```python
from build123d import *

# Parameters (mm, degrees)
SKETCH1_W           = 24
SKETCH1_H           = 16
BOSS_EXTRUDE1_DEPTH = 10
SKETCH2_R           = 4.3
SKETCH2_R_2         = 1.6
CUT_EXTRUDE2_DEPTH  = 11


with BuildPart() as part:
    # Sketch1 → Boss-Extrude1 (new body)
    with BuildSketch(Plane.XY):
        Rectangle(SKETCH1_W, SKETCH1_H)
    extrude(amount=BOSS_EXTRUDE1_DEPTH)

    # Sketch2 → Cut-Extrude2 (cut)
    with BuildSketch(Plane.XY):
        with Locations(Location((0, 0, 0), (0, 0, 180))):
            Circle(SKETCH2_R)
        with Locations(Location((8, 0, 0), (0, 0, 180))):
            Circle(SKETCH2_R_2)
        with Locations(Location((-8, 0, 0), (0, 0, 180))):
            Circle(SKETCH2_R_2)
    extrude(amount=CUT_EXTRUDE2_DEPTH, mode=Mode.SUBTRACT)


solid = part.part
```
The model under review builds one solid part; all positions refer to its coordinate system, in mm. Give positions to 0.01 mm unless a question says otherwise; leave off trailing zeros. Loops run counter-clockwise (first coordinate to the right, second up) from the corner with the lowest first, then second, coordinate; pieces in that order, holes last. Notation, with made-up numbers: (86.5, 71.25) - (132.5, 71.25) arc R16 ccw to (132.5, 102.25) - close; hole circle Ø8 at (70.25, 73). An arc over 180 degrees is marked (long way). Answer as a JSON object with one key per item and string values.
Q1. Add section C-C on y = 0. State the section outline as (x, z) points.
Worked out:
{"outline": "(-12, 0) - (-9.6, 0) - (-9.6, 10) - (-12, 10) - close; (-6.4, 0) - (-4.3, 0) - (-4.3, 10) - (-6.4, 10) - close; (4.3, 0) - (6.4, 0) - (6.4, 10) - (4.3, 10) - close; (9.6, 0) - (12, 0) - (12, 10) - (9.6, 10) - close"}
Q2. Add section B-B on z = 8.5. State the section outline as (x, y) points, plus the area to 3 significant figures.
Worked out:
{"outline": "(-12, -8) - (12, -8) - (12, 8) - (-12, 8) - close; hole circle Ø3.2 at (-8, 0); hole circle Ø8.6 at (0, 0); hole circle Ø3.2 at (8, 0)", "area": "310 mm^2"}
Q3. Add section A-A on x = 0. State the section outline as (y, z) points.
Worked out:
{"outline": "(-8, 0) - (-4.3, 0) - (-4.3, 10) - (-8, 10) - close; (4.3, 0) - (8, 0) - (8, 10) - (4.3, 10) - close"}
Q4. To check wall thickness, follow line 1 along Y through (x, z) = (-8, 5.75); line 2 along Y through (x, z) = (0, 6.5); line 3 along X through (y, z) = (-1, 1.5). State the ranges of each line that lie inside material, in increasing order.
Worked out:
{"line 1": "y = -8 to -1.6, 1.6 to 8", "line 2": "y = -8 to -4.3, 4.3 to 8", "line 3": "x = -12 to -9.25, -6.75 to -4.18, 4.18 to 6.75, 9.25 to 12"}
Q5. Mouldability with a two-part tool opening along Y and no side actions: class faces 1 (the flat face through (-3, 4, 0)), 2 (the cylindrical face through (4.296, -0.189, 4.93)), 3 (the flat face through (0, -8, 5)) as +Y half, -Y half, draft (parallel to the pull), parting line (faces both ways), or undercut.
Worked out:
{"face 1": "draft", "face 2": "undercut", "face 3": "-Y half"}
Q6. Insertion check: pin 1 (2.5 mm diameter, centred on x = 8, y = 0, fed in from -Z). The pin has a flat end and moves straight along its axis. Give the tip position at first contact, or say it passes through.
Worked out:
{"pin 1": "passes through"}
Q7. Add section D-D on y = 2.75. State the section outline as (x, z) points, plus the area to 3 significant figures.
Worked out:
{"outline": "(-12, 0) - (-3.31, 0) - (-3.31, 10) - (-12, 10) - close; (3.31, 0) - (12, 0) - (12, 10) - (3.31, 10) - close", "area": "174 mm^2"}
